```python
from build123d import *

# Parameters (mm, degrees)
SKETCH2_R           = 17.5
SKETCH2_W           = 18.5
SKETCH2_H           = 18.5
BOSS_EXTRUDE1_DEPTH = 2.5
SKETCH4_R           = 1.67
CUT_EXTRUDE1_DEPTH  = 1.15
CIRPATTERN1_COUNT   = 4
SKETCH5_W           = 18.5
SKETCH5_H           = 18.5
SKETCH5_W_2         = 15
SKETCH5_H_2         = 15
BOSS_EXTRUDE2_DEPTH = 0.6
SKETCH10_W          = 1.15
SKETCH10_H          = 6.925
SKETCH10_H_2        = 1.15
SKETCH10_W_2        = 6.925
BOSS_EXTRUDE4_DEPTH = 0.6
FILLET1_R           = 1.15
SKETCH11_R          = 1.5
CUT_EXTRUDE2_DEPTH  = 1.9
CIRPATTERN2_COUNT   = 4


with BuildPart() as part:
    # Sketch2 → Boss-Extrude1 (new body)
    with BuildSketch(Plane(origin=(0, 0, 0), x_dir=(1, 0, 0), z_dir=(0, 1, 0))):
        with Locations(Location((-21.383734207, -0.621346489, 0), (0, 0, 270))):
            Circle(SKETCH2_R)
        with Locations((-21.383734207, -0.621346489)):
            Rectangle(SKETCH2_W, SKETCH2_H, mode=Mode.SUBTRACT)
    extrude(amount=BOSS_EXTRUDE1_DEPTH)

    # Sketch4 → Cut-Extrude1 (cut)
    with BuildSketch(Plane.XZ):
        with Locations(Location((-21.569675845, 15.589648339, 0), (0, 0, 270))):
            Circle(SKETCH4_R)
    cut_extrude1 = extrude(amount=-CUT_EXTRUDE1_DEPTH, mode=Mode.SUBTRACT)

    # CirPattern1: Cut-Extrude1 ×4 about axis
    cirpattern1_axis = Axis((-21.383734207, 0, 0.621346489), (0, 1, 0))
    for i in range(1, CIRPATTERN1_COUNT):
        add(cut_extrude1.rotate(cirpattern1_axis, i * 360 / CIRPATTERN1_COUNT), mode=Mode.SUBTRACT)

    # Sketch5 → Boss-Extrude2 (add)
    with BuildSketch(Plane(origin=(0, 2.5, 0), x_dir=(1, 0, 0), z_dir=(0, 1, 0))):
        with Locations((-21.383734207, -0.621346489)):
            Rectangle(SKETCH5_W, SKETCH5_H)
        with Locations((-21.383734207, -0.621346489)):
            Rectangle(SKETCH5_W_2, SKETCH5_H_2, mode=Mode.SUBTRACT)
    extrude(amount=-BOSS_EXTRUDE2_DEPTH)

    # Sketch10 → Boss-Extrude4 (add)
    with BuildSketch(Plane(origin=(0, 2.5, 0), x_dir=(1, 0, 0), z_dir=(0, 1, 0))):
        with Locations((-21.383734207, 3.416153511)):
            Rectangle(SKETCH10_W, SKETCH10_H)
        with Locations((-21.383734207, -4.658846489)):
            Rectangle(SKETCH10_W, SKETCH10_H)
        with Locations((-21.383734207, -0.621346489)):
            Rectangle(SKETCH10_W, SKETCH10_H_2)
        with Locations((-17.346234207, -0.621346489)):
            Rectangle(SKETCH10_W_2, SKETCH10_H_2)
        with Locations((-25.421234207, -0.621346489)):
            Rectangle(SKETCH10_W_2, SKETCH10_H_2)
    extrude(amount=-BOSS_EXTRUDE4_DEPTH)

    # Fillet1
    fillet1_edges = [part.edges().sort_by_distance(p)[0] for p in [
        (-28.883734207, 2.2, -6.878653511),
        (-28.883734207, 2.2, 8.121346489),
        (-13.883734207, 2.2, 8.121346489),
        (-13.883734207, 2.2, -6.878653511),
        (-28.883734207, 2.2, 0.046346489),
        (-28.883734207, 2.2, 1.196346489),
        (-21.958734207, 2.2, 1.196346489),
        (-21.958734207, 2.2, 8.121346489),
        (-20.808734207, 2.2, 8.121346489),
        (-20.808734207, 2.2, 1.196346489),
        (-13.883734207, 2.2, 1.196346489),
        (-13.883734207, 2.2, 0.046346489),
        (-20.808734207, 2.2, 0.046346489),
        (-20.808734207, 2.2, -6.878653511),
        (-21.958734207, 2.2, -6.878653511),
        (-21.958734207, 2.2, 0.046346489),
    ]]
    fillet(fillet1_edges, radius=FILLET1_R)

    # Sketch11 → Cut-Extrude2 (cut)
    with BuildSketch(Plane.XZ):
        with Locations((-30.133734207, 9.371346489)):
            Circle(SKETCH11_R)
    cut_extrude2 = extrude(amount=-CUT_EXTRUDE2_DEPTH, mode=Mode.SUBTRACT)

    # CirPattern2: Cut-Extrude2 ×4 about axis
    cirpattern2_axis = Axis((-21.383734207, 0, 0.621346489), (0, 1, 0))
    for i in range(1, CIRPATTERN2_COUNT):
        add(cut_extrude2.rotate(cirpattern2_axis, i * 360 / CIRPATTERN2_COUNT), mode=Mode.SUBTRACT)


solid = part.part
```
Model file for the job. Use its own axes, mm. A direction names the side the tool comes from. Give positions to 0.01 mm unless a question says otherwise; leave off trailing zeros. Loops run counter-clockwise (first coordinate to the right, second up) from the corner with the lowest first, then second, coordinate; pieces in that order, holes last. Notation, with made-up numbers: (30, 11) -> (48, 11) arc R35 ccw to (48, 43) -> close; hole circle Ø2 at (-13.75, -3). An arc over 180 degrees is marked (long way). Use CSV: the item, a comma, the result in double quotes. Start each with the question number.
1) Flat gauge pins, fed straight in: pin 1 Ø0.5 at (y, z) = (2.5, -4.5) entering from -X; pin 2 Ø1.5 at (y, z) = (1, 2.5) entering from -X; pin 3 Ø0.7 at (y, z) = (2, 5) entering from -X. Where does each tip first touch, or does it go through?
2) Slice it at B-B on x = -18. Give the cut face in (y, z).
3) Tool access for faces 4 (the flat face through (-33, 0, 0)), 5 (the flat face through (-12.134, 1, 1)), 6 (the cylindrical face through (-28.556, 2.196, 1.542)): list every direction of +Z, -Z, +X, -X, +Y, -Y with a clear straight run to the whole face (end or side of a thin tool).
4) Slice it at A-A on z = 6.5. Give the cut face in (x, y), plus the area to 3 significant figures.
5) Mould opens along X. For faces 1 (the flat face through (-22, 2.5, 0)), 2 (the flat face through (-21, 1, 9.871)), 3 (the cylindrical face through (-38.47, 1.23, -3.17)) say: released by +X, released by -X, zero draft, split by the parting line, or undercut.
6) Slice it at D-D on z = 16.5. Give the cut face in (x, y), plus the area to 3 significant figures.
7) Slice it at C-C on x = -13. Give the cut face in (y, z).
8) Wall check: line 1 (Z direction, x = -31, y = 0.4); line 2 (Z direction, x = -31.5, y = 1); line 3 (Y direction, x = -30, z = -3). Give the ranges that are in metal, low to high.
Computed values:
1,pin 1,"stops at x = -38.19"
1,pin 2,"stops at x = -38.85"
1,pin 3,"stops at x = -38.41"
2,outline,"(0, -16.55) -> (2.5, -16.55) -> (2.5, -6.88) -> (1.9, -6.88) -> (1.9, -8.63) -> (0, -8.63) -> close; (0, 9.87) -> (1.9, 9.87) -> (1.9, 8.12) -> (2.5, 8.12) -> (2.5, 17.79) -> (0, 17.79) -> close; (1.9, 0.05) -> (2.5, 0.05) -> (2.5, 1.2) -> (1.9, 1.2) -> close"
3,face 4,"+Z, -Z, +X, -X, -Y"
3,face 5,"-Y"
3,face 6,"+Y, -Y"
4,outline,"(-37.87, 0) -> (-30.63, 0) -> (-30.63, 1.9) -> (-28.88, 1.9) -> (-28.88, 2.5) -> (-37.87, 2.5) -> close; (-21.96, 1.9) -> (-20.81, 1.9) -> (-20.81, 2.5) -> (-21.96, 2.5) -> close; (-13.88, 1.9) -> (-12.13, 1.9) -> (-12.13, 0) -> (-4.9, 0) -> (-4.9, 2.5) -> (-13.88, 2.5) -> close"
4,area,"39.0 mm^2"
5,face 1,"zero draft"
5,face 2,"undercut"
5,face 3,"split by the parting line"
6,outline,"(-28.74, 0) -> (-22.97, 0) -> (-22.97, 1.15) -> (-20.17, 1.15) -> (-20.17, 0) -> (-14.03, 0) -> (-14.03, 2.5) -> (-28.74, 2.5) -> close"
6,area,"33.6 mm^2"
7,outline,"(0, -14.74) -> (2.5, -14.74) -> (2.5, 15.98) -> (0, 15.98) -> (0, 10.83) -> (1.9, 10.83) -> (1.9, -9.58) -> (0, -9.58) -> close"
8,line 1,"z = -14 to -9.35, -6.9 to 8.15, 10.6 to 15.24"
8,line 2,"z = -13.66 to -8.75, -7.51 to 8.75, 9.99 to 14.9"
8,line 3,"y = 1.9 to 2.5"
